from build123d import *

# Parameters (mm, degrees)
SKETCH_1_W          = 72
SKETCH_1_H          = 25
SKETCH_1_R          = 3.1
EXTRUDE_1_DEPTH     = 4
EXTRUDE_START       = -4
SKETCH_3_W          = 30
SKETCH_3_H          = 5
EXTRUDE_2_DEPTH     = 60
SKETCH_5_W          = 108
SKETCH_5_H          = 11
SKETCH_5_R          = 2.1
EXTRUDE_3_DEPTH     = 5
CUT_EXTRUDE_START   = -5
SKETCH_6_W          = 12
SKETCH_6_H          = 11
CUT_EXTRUDE_1_DEPTH = 2
SKETCH_7_W          = 15
SKETCH_7_H          = 50
CUT_EXTRUDE_2_DEPTH = 88.213817713
EXTRUDE_4_DEPTH     = 2
EXTRUDE_START_2     = -30
EXTRUDE_5_DEPTH     = 2
FILLET_1_R          = 2


with BuildPart() as part:
    # 草图1 → 凸台-拉伸1 (new body)
    with BuildSketch(Plane.XY):
        Rectangle(SKETCH_1_W, SKETCH_1_H)
        with Locations((-27.5, 7.5)):
            Circle(SKETCH_1_R, mode=Mode.SUBTRACT)
        with Locations(Location((27.5, 7.5, 0), (0, 0, 180))):
            Circle(SKETCH_1_R, mode=Mode.SUBTRACT)
    extrude(amount=EXTRUDE_1_DEPTH)

    # 草图3 → 凸台-拉伸2 (add)
    with BuildSketch(Plane.XY.offset(4).offset(EXTRUDE_START)):
        with Locations((0, -10)):
            Rectangle(SKETCH_3_W, SKETCH_3_H)
    extrude(amount=EXTRUDE_2_DEPTH)

    # 草图5 → 凸台-拉伸3 (add, through all)
    with BuildSketch(Plane(origin=(0, -7.5, 0), x_dir=(1, 0, 0), z_dir=(0, 1, 0))):
        with Locations((0, -60)):
            Rectangle(SKETCH_5_W, SKETCH_5_H)
        with Locations(Location((47.5, -60, 0), (0, 0, 270))):
            Circle(SKETCH_5_R, mode=Mode.SUBTRACT)
        with Locations(Location((-47.5, -60, 0), (0, 0, 90))):
            Circle(SKETCH_5_R, mode=Mode.SUBTRACT)
    extrude(amount=-EXTRUDE_3_DEPTH)

    # 草图6 → 切除-拉伸1 (cut)
    with BuildSketch(Plane(origin=(0, -7.5, 0), x_dir=(1, 0, 0), z_dir=(0, 1, 0)).offset(CUT_EXTRUDE_START)):
        with Locations((-48, -60)):
            Rectangle(SKETCH_6_W, SKETCH_6_H)
        with Locations((48, -60)):
            Rectangle(SKETCH_6_W, SKETCH_6_H)
    extrude(amount=CUT_EXTRUDE_1_DEPTH, mode=Mode.SUBTRACT)

    # 草图7 → 切除-拉伸2 (cut, through all)
    with BuildSketch(Plane(origin=(0, -7.5, 0), x_dir=(1, 0, 0), z_dir=(0, 1, 0))):
        with Locations((0, -34)):
            Rectangle(SKETCH_7_W, SKETCH_7_H)
    extrude(amount=-CUT_EXTRUDE_2_DEPTH, mode=Mode.SUBTRACT)

    # 草图8 → 凸台-拉伸4 (add)
    with BuildSketch(Plane.ZY.offset(15)):
        Polygon((4, -7.5), (44, -7.5), (4, 12.5), align=None)
    extrude(amount=-EXTRUDE_4_DEPTH)

    # 草图8<2> → 凸台-拉伸5 (add)
    with BuildSketch(Plane.ZY.offset(15).offset(EXTRUDE_START_2)):
        Polygon((4, -7.5), (44, -7.5), (4, 12.5), align=None)
    extrude(amount=EXTRUDE_5_DEPTH)

    # 圆角1
    fillet_1_edges = [part.edges().sort_by_distance(p)[0] for p in [
        (15, 0, 4),
        (36, 0, 4),
        (36, 0, 0),
        (-36, 0, 0),
        (-36, 0, 4),
        (-15, -10, 54.5),
        (-54, -9, 54.5),
        (-54, -9, 65.5),
        (54, -9, 65.5),
        (54, -9, 54.5),
        (15, -10, 54.5),
        (-15, 0, 4),
        (-42, -11.5, 54.5),
        (42, -11.5, 54.5),
        (42, -11.5, 65.5),
        (-42, -11.5, 65.5),
        (-7.5, -10, 59),
        (-7.5, -10, 9),
        (7.5, -10, 59),
        (7.5, -10, 9),
        (14, -7.5, 44),
        (-14, -7.5, 44),
        (-13, 2.5, 4),
        (13, 2.5, 4),
    ]]
    fillet(fillet_1_edges, radius=FILLET_1_R - 0.0001)  # a hair under: the kernel refuses the full size


solid = part.part
For this review, take the finished solid that the model builds, in its own axes (mm). A direction names the side the tool comes from. Coordinates: 2 decimals unless noted, no trailing zeros. Order: outer loops, then holes, each group sorted by start corner. A loop starts at its lowest first (then second) coordinate and runs counter-clockwise, first axis right, second up. Notation, with made-up numbers: (7.25, -34) -> (18.25, -34) arc R17 ccw to (18.25, -21) -> close; hole circle Ø6 at (3, -2). An arc over 180 degrees is marked (long way). Return JSON: item names as keys, results as strings.
1. The part is to be moulded in two halves that separate along Z. For faces 6 (the cylindrical face through (35.43, 0.18, 0.6)), 7 (the cylindrical face through (45.637, -8.979, 60.969)), 8 (the flat face through (54, -9, 60)), say which applies: +Z half, -Z half, draft (parallel to the pull), parting line (faces both ways), or undercut.
Answer block:
{"face 6": "-Z half", "face 7": "undercut", "face 8": "draft"}
2. For pin 1 Ø12 at (x, y) = (27, -0.5) entering from +Z; pin 2 Ø1.5 at (y, z) = (-10, 29.5) entering from -X; pin 3 Ø12 at (x, z) = (-49.5, 57.5) entering from -Y, all flat-tipped, find the tip position at first contact; note any pin that passes through.
Answer block:
{"pin 1": "z = 4", "pin 2": "x = -15", "pin 3": "y = -10.5"}
3. Machinability: for faces 1 (the flat face through (-42, -12, 60)), 2 (the cylindrical face through (-15.57, -0.17, 4.6)), 3 (the cylindrical face through (6.9, -10.04, 9.57)), 4 (the cylindrical face through (-41.4, -11.49, 64.93)), 5 (the flat face through (42, -12, 60)), which of the approach directions +Z, -Z, +X, -X, +Y, -Y give a long, thin tool a straight path to every point of the face, cutting with its end or side? Answer none if there is none.
Answer block:
{"face 1": "+Z, -Z, -X, -Y", "face 2": "-X, +Y, -Y", "face 3": "+Y, -Y", "face 4": "+Z, -X, -Y", "face 5": "+Z, -Z, +X, -Y"}
4. We need section A-A on z = 35. Write out the cut boundary in (x, y).
Answer block:
{"outline": "(-15, -12.5) -> (-7.5, -12.5) -> (-7.5, -7.5) -> (-13, -7.5) -> (-13, -3) -> (-15, -3) -> close; (7.5, -12.5) -> (15, -12.5) -> (15, -3) -> (13, -3) -> (13, -7.5) -> (7.5, -7.5) -> close"}
5. For line 1 (X direction, y = -8.7, z = 60); line 2 (Z direction, x = -47.5, y = -9.25); line 3 (Y direction, x = 27.5, z = 1.25), list the stretches that pass through material, from the lowest coordinate up. Write a range as from..to.
Answer block:
{"line 1": "-54..-49.6, -45.4..45.4, 49.6..54", "line 2": "54.5..57.9, 62.1..65.5", "line 3": "-12.5..4.4, 10.6..12.5"}
6. We need section D-D on x = 47.5. Write out the cut boundary in (y, z), and give its area (3 significant figures).
Answer block:
{"outline": "(-10.5, 54.5) -> (-7.5, 54.5) -> (-7.5, 57.9) -> (-10.5, 57.9) -> close; (-10.5, 62.1) -> (-7.5, 62.1) -> (-7.5, 65.5) -> (-10.5, 65.5) -> close", "area": "20.4 mm²"}
7. We need section C-C on y = 7.5. State how many separate pieces and enclosed holes the cut face has, and give its area (3 significant figures).
Answer block:
{"separate pieces": "3", "enclosed holes": "0", "area": "278 mm²"}
8. We need section B-B on x = -27.5. Write out the cut boundary in (y, z).
Answer block:
{"outline": "(-12.5, 0) -> (4.4, 0) -> (4.4, 4) -> (-12.5, 4) -> close; (-12.5, 54.5) -> (-7.5, 54.5) -> (-7.5, 65.5) -> (-12.5, 65.5) -> close; (10.6, 0) -> (12.5, 0) -> (12.5, 4) -> (10.6, 4) -> close"}
